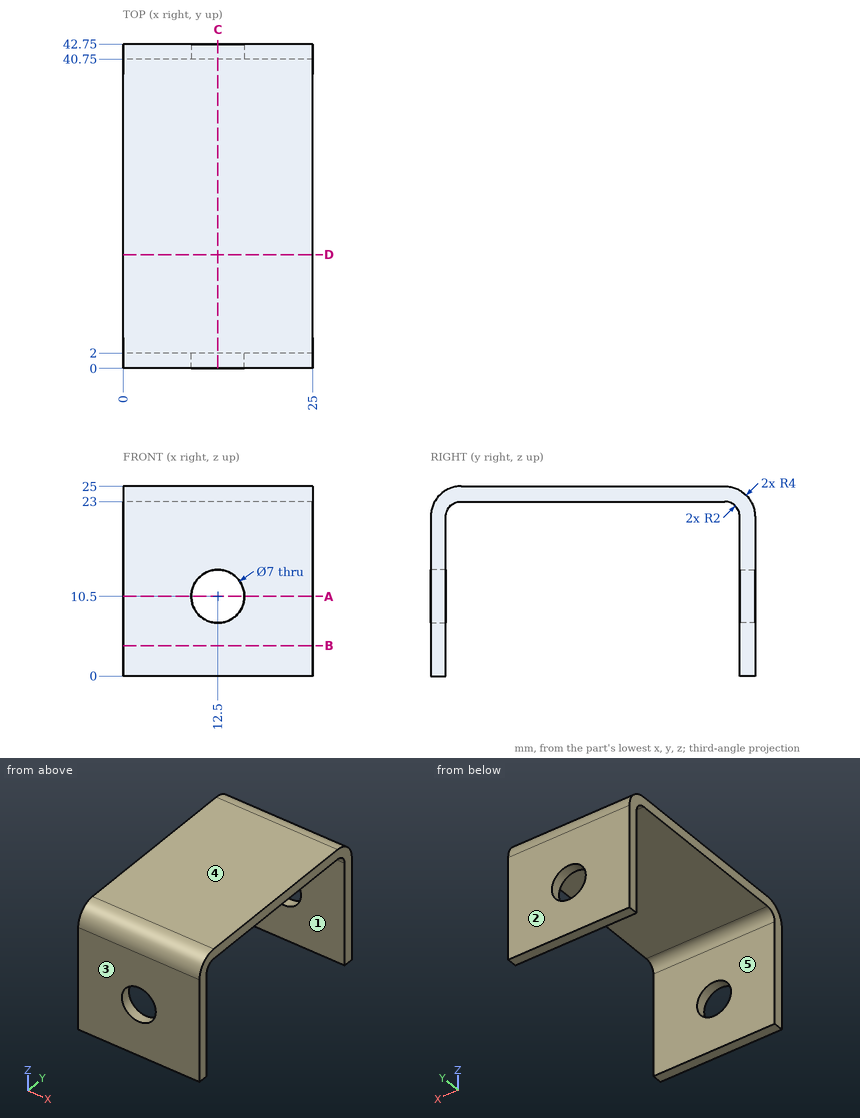
Study the drawing (mm; zero at the part's minimum x, y, z) and answer. A direction names the side the tool comes from. Give positions to 0.01 mm unless a question says otherwise; leave off trailing zeros. Write each loop counter-clockwise with the first axis right and the second up, starting at its lowest first coordinate (ties: lowest second). Pieces come first, ordered by that corner, then holes.
(1) Straight lines are drawn through the part: line 1 (X direction, y = 0.65, z = 10.5); line 2 (Y direction, x = 21, z = 4); line 3 (Z direction, x = 14.5, y = 22.5). For each, find the intervals that lie inside material, in ascending order.
Final values:
line 1: x = 0 to 9, 16 to 25
line 2: y = 0 to 2, 40.75 to 42.75
line 3: z = 23 to 25
(2) The part is cut by section B-B on z = 4. Write down the section's boundary in (x, y), plus the area to 3 significant figures.
Final values:
outline: (0, 0) - (25, 0) - (25, 2) - (0, 2) - close; (0, 40.75) - (25, 40.75) - (25, 42.75) - (0, 42.75) - close
area: 100 mm2
(3) The mould has two halves that part along Y. Classify the marked faces 1, 2 and 3: pulls with the +Y half, pulls with the -Y half, needs draft (parallel to the pull), parting line crosses it, or undercut.
Final values:
face 1: undercut
face 2: pulls with the +Y half
face 3: pulls with the -Y half
(4) The part is cut by section A-A on z = 10.5. Write down the section's boundary in (x, y).
Final values:
outline: (0, 0) - (9, 0) - (9, 2) - (0, 2) - close; (0, 40.75) - (9, 40.75) - (9, 42.75) - (0, 42.75) - close; (16, 0) - (25, 0) - (25, 2) - (16, 2) - close; (16, 40.75) - (25, 40.75) - (25, 42.75) - (16, 42.75) - close
(5) The part is cut by section D-D on y = 15. Write down the section's boundary in (x, z), plus the area to 3 significant figures.
Final values:
outline: (0, 23) - (25, 23) - (25, 25) - (0, 25) - close
area: 50.0 mm2
(6) Flat-ended cylindrical pins translate along their axes: pin 1 Ø3 at (x, z) = (7, 14) entering from -Y; pin 2 Ø3 at (x, y) = (8.5, 35.5) entering from -Z. Find the tip coordinate at first contact, or state that the pin passes through.
Final values:
pin 1: stops at y = 0
pin 2: stops at z = 23
(7) Which of the six approach directions +Z, -Z, +X, -X, +Y, -Y give full straight-line access (tool end or side, diameter ignored) to the marked faces 4 and 5?
Final values:
face 4: +Z, +X, -X, +Y, -Y
face 5: -Z, +X, -X
(8) The part is cut by section C-C on x = 12.5. Write down the section's boundary in (y, z), plus the area to 3 significant figures.
Final values:
outline: (0, 0) - (2, 0) - (2, 7) - (0, 7) - close; (0, 14) - (2, 14) - (2, 21) arc R2 cw to (4, 23) - (38.75, 23) arc R2 cw to (40.75, 21) - (40.75, 14) - (42.75, 14) - (42.75, 21) arc R4 ccw to (38.75, 25) - (4, 25) arc R4 ccw to (0, 21) - close; (40.75, 0) - (42.75, 0) - (42.75, 7) - (40.75, 7) - close
area: 144 mm2
